Input: part model. Units: mm. Frame: model coordinates. A direction names the side the tool comes from. Round coordinates to 2 decimals unless told otherwise and drop trailing zeros. Loops run counter-clockwise (first coordinate to the right, second up) from the corner with the lowest first, then second, coordinate; pieces in that order, holes last. Notation, with made-up numbers: M 31,-16.75 L 58,-16.75 A17 ccw 58,-8.75 Z; hole C -35,58 d5. An arc over 180 degrees is marked long. Return JSON: item names as keys, results as strings. Group by question number.
1) Access query for faces 1 (the face through (185, -157, -23)), 2 (the face through (7.5, 0, -23)), 3 (the face through (-73, -151, -44)). Directions: +Z, -Z, +X, -X, +Y, -Y. A direction counts if a zero-diameter tool reaches every point of the face in a straight line with its end or side. Return the directions, or none.
2) Material intervals for line 1 (X direction, y = -149.5, z = -45.1); line 2 (Y direction, x = 0, z = -44.65); line 3 (X direction, y = -149, z = -45), sorted ascending. Write a range as from..to.
3) Section C-C (x = -49). Output: boundary loops of the cut face in (y, z).
4) Section A-A (z = -4). Output: boundary loops of the cut face in (x, y).
5) Contact query for flat-ended pins moving along their axis: P1, Ø17.5, axis at x = 0, y = 0, coming from the +Z side; P2, Ø3.5, axis at x = 1.5, y = 2, coming from the +Z side; P3, Ø16.5, axis at x = -0.5, z = -21, coming from the +Y side; P4, Ø2.5, axis at y = 65, z = 2, coming from the +X side. Output: stop coordinate, or through.
6) Mould query, pull axis Y, two halves, no side actions, for faces 4 (the face through (53, -62, 0)), 5 (the face through (-3, 0, -44)), 6 (the face through (-75, -142, -23)). Classes: +Y half, -Y half, draft (parallel to the pull), parting line (faces both ways), or undercut.
7) Section B-B (y = 55.5). Output: boundary loops of the cut face in (x, z), plus the area to 4 significant figures.
Autodesk Inventor part; units mm, degrees
ref_plane "YZ Plane" through (0, 0, 0) normal (1, 0, 0) x (0, 1, 0)
ref_plane "XZ Plane" through (0, 0, 0) normal (0, 1, 0) x (-1, 0, 0)
ref_plane "XY Plane" through (0, 0, 0) normal (0, 0, 1) x (1, 0, 0)
sketch "Sketch1" plane through (0, 0, 0) normal (0, 0, 1) x (1, 0, 0)
  circle A0 centre (0, 0) radius 2.5
  circle A1 centre (109.2883, 0) radius 2.5
  line L0 (-82.8559, 30) -> (192.1441, 30)
  line L1 (192.1441, 30) -> (192.1441, -175)
  line L2 (192.1441, -175) -> (-82.8559, -175)
  line L3 (-82.8559, -175) -> (-82.8559, 30)
  line L4 (0, 0) -> (109.2883, 0) construction
  point P0 (54.6441, 0)
  point P1 (54.6441, 30)
  dimension "d0" = 5
  dimension "d1" = 5
  dimension "d2" = 109.2883
  dimension "d3" = 275
  dimension "d4" = 30
  dimension "d5" = 175
extrude "Extrusion1" add sketch "Sketch1" along normal blind 3
sketch "Sketch4" plane through (0, 0, 0) normal (0, 0, -1) x (-1, 0, 0)
  circle A0 centre (-109.2883, 0) radius 2.5
  line L0 (-116.7883, -7.5) -> (-101.7883, -7.5)
  line L1 (-101.7883, -7.5) -> (-101.7883, 7.5)
  line L2 (-101.7883, 7.5) -> (-116.7883, 7.5)
  line L3 (-116.7883, 7.5) -> (-116.7883, -7.5)
  circle A1 centre (-109.2883, 0) radius 2.5
  line L4 (-116.7883, -7.5) -> (-101.7883, 7.5) construction
  line L5 (-101.7883, -7.5) -> (-116.7883, 7.5) construction
  line L6 (7.5, -7.5) -> (-7.5, -7.5)
  line L7 (-7.5, -7.5) -> (-7.5, 7.5)
  line L8 (-7.5, 7.5) -> (7.5, 7.5)
  line L9 (7.5, 7.5) -> (7.5, -7.5)
  circle A2 centre (0, 0) radius 2.5
  line L10 (7.5, -7.5) -> (-7.5, 7.5) construction
  line L11 (-7.5, -7.5) -> (7.5, 7.5) construction
  dimension "d14" = 15
  dimension "d15" = 15
  dimension "d16" = 15
  dimension "d17" = 15
extrude "Extrusion4" add sketch "Sketch4" along normal blind 47
sketch "Sketch5" plane through (0, 0, 3) normal (0, 0, 1) x (1, 0, 0)
  circle A0 centre (0, 0) radius 2.5
  circle A1 centre (109.2883, 0) radius 2.5
  circle A2 centre (0, 0) radius 5.5
  circle A3 centre (109.2883, 0) radius 5.5
  dimension "d20" = 11
  dimension "d21" = 11
extrude "Extrusion5" cut sketch "Sketch5" against normal blind 47
sketch "Sketch6" plane through (0, 0, 0) normal (0, 0, -1) x (-1, 0, 0)
  line L0 (-192.1441, 30) -> (-192.1441, -175)
  line L1 (-192.1441, -157) -> (-177.1441, -157)
  line L2 (-177.1441, -157) -> (-177.1441, -142)
  line L3 (-177.1441, -142) -> (-192.1441, -142)
  line L4 (-192.1441, -142) -> (-192.1441, -157)
  line L5 (82.8559, -175) -> (82.8559, 30)
  line L6 (82.8559, -157) -> (67.8559, -157)
  line L7 (67.8559, -157) -> (67.8559, -142)
  line L8 (67.8559, -142) -> (82.8559, -142)
  line L9 (82.8559, -142) -> (82.8559, -157)
  line L10 (-192.1441, -175) -> (82.8559, -175)
  point P0 (0, 0)
  dimension "d24" = 15
  dimension "d25" = 15
  dimension "d26" = 15
  dimension "d27" = 15
  dimension "d28" = 18
extrude "Extrusion6" add sketch "Sketch6" along normal blind 47
sketch "Sketch7" plane through (0, 0, 3) normal (0, 0, 1) x (1, 0, 0)
  line L0 (-10.3559, 30) -> (-82.8559, 30)
  line L1 (-82.8559, 30) -> (-10.3559, 30)
  line L2 (-10.3559, 30) -> (-10.3559, 110)
  line L3 (-10.3559, 110) -> (-82.8559, 110)
  line L4 (-82.8559, 110) -> (-82.8559, 30)
  line L5 (-82.8559, 30) -> (-82.8559, -175)
  point P0 (0, 0)
  dimension "d31" = 80
  dimension "d42" = 72.5
extrude "Extrusion7" add sketch "Sketch7" against normal blind 3
sketch "Sketch8" plane through (0, 0, -47) normal (0, 0, -1) x (-1, 0, 0)
  line L0 (-192.1441, -157) -> (-177.1441, -157)
  line L1 (-177.1441, -157) -> (-177.1441, -142)
  line L2 (-177.1441, -142) -> (-192.1441, -142)
  line L3 (-192.1441, -142) -> (-192.1441, -157)
  line L4 (82.8559, -157) -> (82.8559, -142)
  line L5 (82.8559, -142) -> (67.8559, -142)
  line L6 (67.8559, -142) -> (67.8559, -157)
  line L7 (67.8559, -157) -> (82.8559, -157)
  circle A0 centre (-184.6441, -149.5) radius 2.5
  circle A1 centre (75.3559, -149.5) radius 2.5
  point P0 (0, 0)
  point P1 (75.3559, -157)
  point P2 (-184.6441, -157)
  point P3 (-177.1441, -149.5)
  point P4 (67.8559, -149.5)
  dimension "d34" = 5
  dimension "d35" = 5
extrude "Extrusion8" cut sketch "Sketch8" against normal through all contours A0 | A1
sketch "Sketch9" plane through (0, 0, 3) normal (0, 0, 1) x (1, 0, 0)
  circle A0 centre (-75.3559, -149.5) radius 2.5
  circle A1 centre (184.6441, -149.5) radius 2.5
  circle A2 centre (-75.3559, -149.5) radius 5.5
  circle A3 centre (184.6441, -149.5) radius 5.5
  point P0 (0, 0)
  dimension "d38" = 11
  dimension "d39" = 11
extrude "Extrusion9" cut sketch "Sketch9" against normal blind 47
sketch "Sketch10" plane through (0, 0, 3) normal (0, 0, 1) x (1, 0, 0)
  line L0 (192.1441, 30) -> (-10.3559, 30)
  line L1 (-10.3559, 30) -> (-10.3559, 110)
  line L2 (-10.3559, 30) -> (192.1441, 30)
  line L3 (-10.3559, 110) -> (-10.3559, 30)
  line L4 (192.1441, 30) -> (-10.3559, 30)
  line L5 (-10.3559, 30) -> (-10.3559, 50)
  line L6 (-10.3559, 50) -> (192.1441, 50)
  line L7 (192.1441, 50) -> (192.1441, 30)
  point P0 (0, 0)
  dimension "d43" = 20
extrude "Extrusion10" add sketch "Sketch10" against normal blind 3
properties part number "BP013" material "ABS Plastic"
Returned:
{
 "1": {"face 1": "-Z, +X, -X, -Y", "face 2": "-Z, +Y, -Y", "face 3": "+Z"},
 "2": {"line 1": "x = -82.86..-77.86, -72.86..-67.86, 177.14..182.14, 187.14..192.14", "line 2": "y = -7.5..-2.5, 2.5..7.5", "line 3": "x = -82.86..-77.81, -72.91..-67.86, 177.14..182.19, 187.09..192.14"},
 "3": {"outline": "M -175,0 L 110,0 L 110,3 L -175,3 Z"},
 "4": {"outline": "M -82.86,-157 L -67.86,-157 L -67.86,-142 L -82.86,-142 Z; M -7.5,-7.5 L 7.5,-7.5 L 7.5,7.5 L -7.5,7.5 Z; M 101.79,-7.5 L 116.79,-7.5 L 116.79,7.5 L 101.79,7.5 Z; M 177.14,-157 L 192.14,-157 L 192.14,-142 L 177.14,-142 Z; hole C -75.36,-149.5 d11; hole C 0,0 d11; hole C 109.29,0 d11; hole C 184.64,-149.5 d11"},
 "5": {"P1": "stops at z = 3", "P2": "stops at z = -44", "P3": "stops at y = 7.5", "P4": "stops at x = -10.36"},
 "6": {"face 4": "draft", "face 5": "undercut", "face 6": "+Y half"},
 "7": {"outline": "M -82.86,0 L -10.36,0 L -10.36,3 L -82.86,3 Z", "area": "217.5 mm^2"}
}
